from build123d import *

# Parameters (mm, degrees)
SKETCH1_R                = 133.35
SKETCH1_R_2              = 4
BOSS_EXTRUDE1_DEPTH      = 4.445
BOSS_EXTRUDE1_DEPTH_BACK = 4.445


with BuildPart() as part:
    # Sketch1 → Boss-Extrude1 (new body, two sides)
    with BuildSketch(Plane.XY) as boss_extrude1_sk:
        Circle(SKETCH1_R)
        with Locations((0, 69.85)):
            Circle(SKETCH1_R_2, mode=Mode.SUBTRACT)
        with Locations((60.491874454, 34.925)):
            Circle(SKETCH1_R_2, mode=Mode.SUBTRACT)
        with Locations((60.491874454, -34.925)):
            Circle(SKETCH1_R_2, mode=Mode.SUBTRACT)
        with Locations((0, -69.85)):
            Circle(SKETCH1_R_2, mode=Mode.SUBTRACT)
        with Locations((-60.491874454, -34.925)):
            Circle(SKETCH1_R_2, mode=Mode.SUBTRACT)
        with Locations((-60.491874454, 34.925)):
            Circle(SKETCH1_R_2, mode=Mode.SUBTRACT)
        with BuildLine():
            Line((14.785375278, 74.430875165), (10.324543782, 61.882634395))
            ThreePointArc((10.324543782, 61.882634395), (5.179957882, 62.523792914), (0, 62.738))
            ThreePointArc((0, 62.738), (-5.179957882, 62.523792914), (-10.324543782, 61.882634395))
            Line((-10.324543782, 61.882634395), (-14.785375278, 74.430875165))
            ThreePointArc((-14.785375278, 74.430875165), (-23.474698759, 83.741706154), (-36.210304588, 83.757843464))
            ThreePointArc((-36.210304588, 83.757843464), (-45.625, 79.024818095), (-54.431267912, 73.237965383))
            ThreePointArc((-54.431267912, 73.237965383), (-60.785095506, 62.200538548), (-57.06634108, 50.019948178))
            Line((-57.06634108, 50.019948178), (-48.429661548, 39.882634395))
            ThreePointArc((-48.429661548, 39.882634395), (-51.557214064, 35.747871573), (-54.332701783, 31.369))
            ThreePointArc((-54.332701783, 31.369), (-56.737171945, 26.775921341), (-58.75420533, 22))
            Line((-58.75420533, 22), (-71.851716358, 24.410926987))
            ThreePointArc((-71.851716358, 24.410926987), (-84.259794265, 21.541167606), (-90.641572499, 10.51987808))
            ThreePointArc((-90.641572499, 10.51987808), (-91.25, 0), (-90.641572499, -10.51987808))
            ThreePointArc((-90.641572499, -10.51987808), (-84.259794265, -21.541167606), (-71.851716358, -24.410926987))
            Line((-71.851716358, -24.410926987), (-58.75420533, -22))
            ThreePointArc((-58.75420533, -22), (-56.737171945, -26.775921341), (-54.332701783, -31.369))
            ThreePointArc((-54.332701783, -31.369), (-51.557214064, -35.747871573), (-48.429661548, -39.882634395))
            Line((-48.429661548, -39.882634395), (-57.06634108, -50.019948178))
            ThreePointArc((-57.06634108, -50.019948178), (-60.785095506, -62.200538548), (-54.431267912, -73.237965383))
            ThreePointArc((-54.431267912, -73.237965383), (-45.625, -79.024818095), (-36.210304588, -83.757843464))
            ThreePointArc((-36.210304588, -83.757843464), (-23.474698759, -83.741706154), (-14.785375278, -74.430875165))
            Line((-14.785375278, -74.430875165), (-10.324543782, -61.882634395))
            ThreePointArc((-10.324543782, -61.882634395), (-5.179957882, -62.523792914), (0, -62.738))
            ThreePointArc((0, -62.738), (5.179957882, -62.523792914), (10.324543782, -61.882634395))
            Line((10.324543782, -61.882634395), (14.785375278, -74.430875165))
            ThreePointArc((14.785375278, -74.430875165), (23.474698759, -83.741706154), (36.210304588, -83.757843464))
            ThreePointArc((36.210304588, -83.757843464), (45.625, -79.024818095), (54.431267912, -73.237965383))
            ThreePointArc((54.431267912, -73.237965383), (60.785095506, -62.200538548), (57.06634108, -50.019948178))
            Line((57.06634108, -50.019948178), (48.429661548, -39.882634395))
            ThreePointArc((48.429661548, -39.882634395), (51.557214064, -35.747871573), (54.332701783, -31.369))
            ThreePointArc((54.332701783, -31.369), (56.737171945, -26.775921341), (58.75420533, -22))
            Line((58.75420533, -22), (71.851716358, -24.410926987))
            ThreePointArc((71.851716358, -24.410926987), (84.259794265, -21.541167606), (90.641572499, -10.51987808))
            ThreePointArc((90.641572499, -10.51987808), (91.25, 0), (90.641572499, 10.51987808))
            ThreePointArc((90.641572499, 10.51987808), (84.259794265, 21.541167606), (71.851716358, 24.410926987))
            Line((71.851716358, 24.410926987), (58.75420533, 22))
            ThreePointArc((58.75420533, 22), (56.737171945, 26.775921341), (54.332701783, 31.369))
            ThreePointArc((54.332701783, 31.369), (51.557214064, 35.747871573), (48.429661548, 39.882634395))
            Line((48.429661548, 39.882634395), (57.06634108, 50.019948178))
            ThreePointArc((57.06634108, 50.019948178), (60.785095506, 62.200538548), (54.431267912, 73.237965383))
            ThreePointArc((54.431267912, 73.237965383), (45.625, 79.024818095), (36.210304588, 83.757843464))
            ThreePointArc((36.210304588, 83.757843464), (23.474698759, 83.741706154), (14.785375278, 74.430875165))
        make_face(mode=Mode.SUBTRACT)
    extrude(amount=BOSS_EXTRUDE1_DEPTH)
    extrude(boss_extrude1_sk.sketch, amount=-BOSS_EXTRUDE1_DEPTH_BACK)

    # Sketch2 → Cut-Revolve1 (revolve, cut)
    with BuildSketch(Plane(origin=(0, 0, 0), x_dir=(0, 0, -1), z_dir=(1, 0, 0))):
        Polygon((0, 0), (-8.445, 133.35), (-26.557438236, 133.35), (-26.557438236, 0), align=None)
    revolve(axis=Axis((0, 0, 33.831792396), (0, 0, -1)), mode=Mode.SUBTRACT)


solid = part.part
Work out the finished part from the listing and answer in its coordinate system (mm). A direction names the side the tool comes from. Give positions to 0.01 mm unless a question says otherwise; leave off trailing zeros. Order: outer loops, then holes, each group sorted by start corner. A loop starts at its lowest first (then second) coordinate and runs counter-clockwise, first axis right, second up. Notation, with made-up numbers: M 35.5,25 L 57.5,25 A12 ccw 57.5,34 Z; hole C 40.25,60.25 d7. An arc over 180 degrees is marked long. Return JSON: item names as keys, results as strings.
Q1. Find section C-C, the plane x = 0. Write down the section's boundary in (y, z) (3 decimals), and give its area (3 significant figures).
Answer below:
{"outline": "M -133.35,-4.445 L -73.85,-4.445 L -73.85,4.445 L -133.35,4.445 Z; M -65.85,-4.445 L -62.738,-4.445 L -62.738,3.973 L -65.85,4.17 Z; M 62.738,-4.445 L 65.85,-4.445 L 65.85,4.17 L 62.738,3.973 Z; M 73.85,-4.445 L 133.35,-4.445 L 133.35,4.445 L 73.85,4.445 Z", "area": "1,110 mm^2"}
Q2. Find section D-D, the plane z = -0.75. State how many separate pieces and enclosed holes the cut face has, and give its area (3 significant figures).
Answer below:
{"separate pieces": "1", "enclosed holes": "7", "area": "35,300 mm^2"}
Q3. Each of these flat-tipped pins is pushed along its axis until it touches: pin 1 (6.5 mm diameter, centred on x = 0, y = 69.85, fed in from -Z); pin 2 (1.5 mm diameter, centred on y = 106.5, z = -1.5, fed in from -X); pin 3 (1.5 mm diameter, centred on x = -37, z = 3.5, fed in from -Y); pin 4 (1.5 mm diameter, centred on y = 52, z = -1, fed in from +X). Where does it stop, or does it pass through?
Answer below:
{"pin 1": "passes through", "pin 2": "stops at x = -81.24", "pin 3": "stops at y = -128.33", "pin 4": "stops at x = 123.11"}
Q4. Find section A-A, the plane y = 0. Write down the section's boundary in (x, z) (3 decimals), and give its area (3 significant figures).
Answer below:
{"outline": "M -133.35,-4.445 L -91.25,-4.445 L -91.25,4.445 L -133.35,4.445 Z; M 91.25,-4.445 L 133.35,-4.445 L 133.35,4.445 L 91.25,4.445 Z", "area": "749 mm^2"}
Q5. Find the intervals of material crossed by line 1 along Y through (x, z) = (2, 3.5) (3 decimals); line 2 along X through (y, z) = (25, 0.75); line 3 along X through (y, z) = (-49, 1.75), in increasing order. Write a range as [from, to].
Answer below:
{"line 1": "y = [-133.335, -73.314], [-66.386, -62.706], [62.706, 66.386], [73.314, 133.335]", "line 2": "x = [-130.99, -57.54], [57.54, 130.99]", "line 3": "x = [-124.02, -56.2], [56.2, 124.02]"}
Q6. Find section B-B, the plane x = -81.5. Write down the section's boundary in (y, z) (3 decimals).
Answer below:
{"outline": "M -105.546,-4.445 L -23.181,-4.445 L -23.181,4.445 L -105.546,4.445 Z; M 23.181,-4.445 L 105.546,-4.445 L 105.546,4.445 L 23.181,4.445 Z"}
Q7. Which of the six approach directions +Z, -Z, +X, -X, +Y, -Y give full straight-line access (tool end or side, diameter ignored) to faces 3 (the face through (84.41, 21.43, 0.06)), 4 (the face through (-56.97, 32.7, 4.16))?
Answer below:
{"face 3": "+Z, -Z", "face 4": "+Z"}
Q8. The mould has two halves that part along Y. Classify faces 1 (the face through (-60.763, 62.383, 0.062)), 2 (the face through (127.192, 40.055, 0.062)): pulls with the +Y half, pulls with the -Y half, needs draft (parallel to the pull), parting line crosses it, or undercut.
Answer below:
{"face 1": "undercut", "face 2": "parting line crosses it"}
